Work out the finished part from the listing and answer in its coordinate system (mm). A direction names the side the tool comes from. Round coordinates to 2 decimals unless told otherwise and drop trailing zeros. Order: outer loops, then holes, each group sorted by start corner. A loop starts at its lowest first (then second) coordinate and runs counter-clockwise, first axis right, second up. Notation, with made-up numbers: (6.5, 85.25) - (18.5, 85.25) arc R26 ccw to (18.5, 116.25) - close; hole circle Ø6 at (-12, 1.25). An arc over 180 degrees is marked (long way). One line per question, with ' | ' between items. Start each with the question number.
Autodesk Fusion 360 part; units mm, degrees
sketch "Skizze5" plane through (0, 0, 0) normal (0, 1, 0) x (1, 0, 0)
  line L0 (3, 0) -> (97, 0)
  line L1 (80, -66) -> (80, -68.7)
  line L2 (69.2, -75) -> (30.8, -75)
  line L3 (20, -68.7) -> (20, -66)
  line L4 (97, -65) -> (81, -65)
  line L5 (19, -65) -> (3, -65)
  line L6 (20, -68.7) -> (30.8, -75)
  line L7 (80, -68.7) -> (69.2, -75)
  arc A0 (20, -66) -> (19, -65) centre (19, -66) ccw
  arc A1 (81, -65) -> (80, -66) centre (81, -66) ccw
  arc A2 (0, -62) -> (3, -65) centre (3, -62) ccw
  arc A3 (97, -65) -> (100, -62) centre (97, -62) ccw
  arc A4 (100, -3) -> (97, 0) centre (97, -3) ccw
  arc A5 (3, 0) -> (0, -3) centre (3, -3) ccw
  line L8 (0, -46) -> (2, -46)
  line L9 (3, -45) -> (3, -15)
  line L10 (2, -14) -> (0, -14)
  line L11 (0, -62) -> (0, -46)
  line L12 (0, -14) -> (0, -3)
  arc A6 (2, -46) -> (3, -45) centre (2, -45) ccw
  arc A7 (3, -15) -> (2, -14) centre (2, -15) ccw
  line L13 (100, -46) -> (98, -46)
  line L14 (97, -45) -> (97, -15)
  line L15 (98, -14) -> (100, -14)
  line L16 (100, -3) -> (100, -14)
  line L17 (100, -46) -> (100, -62)
  arc A8 (97, -45) -> (98, -46) centre (98, -45) ccw
  arc A9 (98, -14) -> (97, -15) centre (98, -15) ccw
  point P0 (100, 0)
  point P1 (0, -65)
  point P2 (20, -65)
  point P3 (80, -65)
  point P4 (3, -46)
  point P5 (3, -14)
  point P6 (97, -46)
  point P7 (97, -14)
  dimension "d46" = 100
  dimension "d47" = 65
  dimension "d48" = 20
  dimension "d49" = 20
  dimension "d51" = 3.7
  dimension "d52" = 3.7
  dimension "d53" = 10.8
  dimension "d54" = 10.8
  dimension "d55" = 10
  dimension "d56" = 1
  dimension "d57" = 1
  dimension "d58" = 3
  dimension "d59" = 3
  dimension "d60" = 3
  dimension "d61" = 3
  dimension "d62" = 3
  dimension "d63" = 32
  dimension "d64" = 14
  dimension "d65" = 1
  dimension "d66" = 1
  dimension "d67" = 32
  dimension "d68" = 14
  dimension "d69" = 3
  dimension "d70" = 1
  dimension "d71" = 1
extrude "Extrusion1" add sketch "Skizze5" along normal blind 1.6
sketch "Skizze6" plane through (0, 0, 0) normal (0, -1, 0) x (1, 0, 0)
  arc A0 (97, 0) -> (100, 3) centre (97, 3) ccw
  line L0 (100, 3) -> (100, 14)
  line L1 (100, 14) -> (98, 14)
  arc A1 (97, 15) -> (98, 14) centre (98, 15) ccw
  line L2 (97, 15) -> (97, 45)
  arc A2 (98, 46) -> (97, 45) centre (98, 45) ccw
  line L3 (98, 46) -> (100, 46)
  line L4 (100, 46) -> (100, 62)
  arc A3 (100, 62) -> (97, 65) centre (97, 62) ccw
  line L5 (97, 65) -> (81, 65)
  arc A4 (80, 66) -> (81, 65) centre (81, 66) ccw
  line L6 (80, 66) -> (80, 68.7)
  line L7 (80, 68.7) -> (69.2, 75)
  line L8 (69.2, 75) -> (30.8, 75)
  line L9 (30.8, 75) -> (20, 68.7)
  line L10 (20, 68.7) -> (20, 66)
  arc A5 (19, 65) -> (20, 66) centre (19, 66) ccw
  line L11 (19, 65) -> (3, 65)
  arc A6 (3, 65) -> (0, 62) centre (3, 62) ccw
  line L12 (0, 62) -> (0, 46)
  line L13 (0, 46) -> (2, 46)
  arc A7 (3, 45) -> (2, 46) centre (2, 45) ccw
  line L14 (3, 45) -> (3, 15)
  arc A8 (2, 14) -> (3, 15) centre (2, 15) ccw
  line L15 (2, 14) -> (0, 14)
  line L16 (0, 14) -> (0, 3)
  arc A9 (0, 3) -> (3, 0) centre (3, 3) ccw
  line L17 (3, 0) -> (97, 0)
  circle A10 centre (50, 68.5) radius 3
  line L18 (32, 65.5) -> (40, 65.5)
  arc A11 (40, 65.5) -> (40, 71.5) centre (40, 68.5) ccw
  line L19 (40, 71.5) -> (32, 71.5)
  arc A12 (32, 71.5) -> (32, 65.5) centre (32, 68.5) ccw
  line L20 (32, 68.5) -> (40, 68.5) construction
  line L21 (68, 71.5) -> (60, 71.5)
  arc A13 (60, 71.5) -> (60, 65.5) centre (60, 68.5) ccw
  line L22 (60, 65.5) -> (68, 65.5)
  arc A14 (68, 65.5) -> (68, 71.5) centre (68, 68.5) ccw
  line L23 (68, 68.5) -> (60, 68.5) construction
  point P0 (36, 68.5)
  point P1 (64, 68.5)
  dimension "d77" = 50
  dimension "d78" = 68.5
  dimension "d79" = 6
  dimension "d88" = 8
  dimension "d89" = 8
  dimension "d90" = 6
  dimension "d91" = 6
  dimension "d92" = 68.5
  dimension "d93" = 68.5
  dimension "d94" = 36
  dimension "d95" = 36
extrude "Extrusion5" cut sketch "Skizze6" against normal blind 1.6 contours A10 | L18 A11 L19 A12 | L21 A13 L22 A14
1) Flat-ended cylindrical pins translate along their axes: pin 1 (0.5 mm diameter, centred on x = 1.5, y = 1, fed in from +Z); pin 2 (0.8 mm diameter, centred on x = 37.5, y = 1, fed in from -Z); pin 3 (5 mm diameter, centred on x = 50, z = 68.5, fed in from -Y); pin 4 (0.5 mm diameter, centred on x = 1, y = 0.5, fed in from -Z). Find the tip coordinate at first contact, or state that the pin passes through.
2) For faces 1 (the cylindrical face through (43, 0.8, 68.4)), 2 (the flat face through (49, 0, 37)), determine the directions among +Z, -Z, +X, -X, +Y, -Y from which every point of the face is accessible in a straight line to the end or side of a thin tool.
3) Section D-D on x = 9.5 is taken. Give the vertices of the cut face in (y, z), and give its area (3 significant figures).
4) Straight lines are drawn through the part: line 1 (Z direction, x = 37, y = 1.3); line 2 (X direction, y = 0.5, z = 67); line 3 (X direction, y = 1.35, z = 26.5). For each, find the intervals that lie inside material, in ascending order.
5) Section C-C on z = 41 is taken. Give the vertices of the cut face in (x, y).
6) Section B-B on y = 0.95 is taken. Give the number of separate pieces and of enclosed holes in the cut face, and give its area (3 significant figures).
7) Determine the mould class of faces 3 (the flat face through (25.324, 0.789, 71.806)), 4 (the flat face through (49, 1.6, 37)), 5 (the cylindrical face through (29, 0.8, 68.6)) for opening direction X: released by +X, released by -X, zero draft, split by the parting line, or undercut.
8) Section A-A on x = 38.5 is taken. Give the vertices of the cut face in (y, z).
Recorded:
1) pin 1: stops at z = 64.73 | pin 2: stops at z = 0 | pin 3: passes through | pin 4: stops at z = 0.56
2) face 1: +Y, -Y | face 2: +Z, -Z, +X, -X, -Y
3) outline: (0, 0) - (1.6, 0) - (1.6, 65) - (0, 65) - close | area: 104 mm²
4) line 1: z = 0 to 65.5, 71.5 to 75 | line 2: x = 20 to 29.4, 42.6 to 47.4, 52.6 to 57.4, 70.6 to 80 | line 3: x = 3 to 97
5) outline: (3, 0) - (97, 0) - (97, 1.6) - (3, 1.6) - close
6) separate pieces: 1 | enclosed holes: 3 | area: 6,650 mm²
7) face 3: released by -X | face 4: zero draft | face 5: undercut
8) outline: (0, 0) - (1.6, 0) - (1.6, 65.5) - (0, 65.5) - close; (0, 71.5) - (1.6, 71.5) - (1.6, 75) - (0, 75) - close
